```python
from build123d import *

# Parameters (mm, degrees)
BOSS_EXTRUDE1_DEPTH = 15
SKETCH2_R           = 7.490706033
BOSS_EXTRUDE2_DEPTH = 5
SKETCH3_R           = 8.44094948
BOSS_EXTRUDE3_DEPTH = 7
FILLET1_R           = 1


with BuildPart() as part:
    # Sketch1 → Boss-Extrude1 (new body)
    with BuildSketch(Plane(origin=(0, 0, 0), x_dir=(1, 0, 0), z_dir=(0, 1, 0))):
        with BuildLine():
            Line((-17.967290282, 0), (-45.431439127, 0))
            ThreePointArc((-45.431439127, 0), (-58.787226235, 13.355787108), (-45.431439127, 26.711574216))
            Line((-45.431439127, 26.711574216), (5.45092281, 18.253380544))
            ThreePointArc((5.45092281, 18.253380544), (25.659892843, 17.20031813), (45.593289448, 20.689029929))
            Line((45.593289448, 20.689029929), (45.940338636, 20.791055963))
            Line((45.940338636, 20.791055963), (45.352375673, 22.791055963))
            ThreePointArc((45.352375673, 22.791055963), (25.570805515, 18.868293737), (5.45092281, 20.242666786))
            Line((5.45092281, 20.242666786), (-45.495890395, 28.711574216))
            ThreePointArc((-45.495890395, 28.711574216), (-62.583598174, 18.547920568), (-55.423692083, 0))
            Line((-55.423692083, 0), (-125.431439127, 0))
            Line((-125.431439127, 0), (-157.707883989, -16.232049306))
            Line((-157.707883989, -16.232049306), (-156.809303927, -18.01882122))
            Line((-156.809303927, -18.01882122), (-124.532859065, -1.786771914))
            Line((-124.532859065, -1.786771914), (-17.068710221, -1.786771914))
            ThreePointArc((-17.068710221, -1.786771914), (1.299435065, -3.480980646), (19.190909572, -7.970328534))
            Line((19.190909572, -7.970328534), (30.410309542, -11.40707822))
            Line((30.410309542, -11.40707822), (30.996087081, -9.494785179))
            Line((30.996087081, -9.494785179), (17.179362085, -5.262417546))
            ThreePointArc((17.179362085, -5.262417546), (-0.198073846, -1.322896281), (-17.967290282, 0))
        make_face()
    extrude(amount=BOSS_EXTRUDE1_DEPTH)

    # Sketch2 → Boss-Extrude2 (add)
    with BuildSketch(Plane(origin=(-132.388101561, 0, 66.578899913), x_dir=(0.4492900307338926, 0, 0.8933859570662267), z_dir=(-0.8933859570662267, 0, 0.4492900307338926))):
        with Locations(Location((-55.356167213, 7.508040546, 0), (0, 0, 97.663545488))):
            Circle(SKETCH2_R)
    extrude(amount=BOSS_EXTRUDE2_DEPTH)

    # Sketch3 → Boss-Extrude3 (add)
    with BuildSketch(Plane(origin=(-136.855031347, 0, 68.825350067), x_dir=(0.4492900307338926, 0, 0.8933859570662267), z_dir=(-0.8933859570662267, 0, 0.4492900307338926))):
        with Locations((-55.356167213, 7.508040546)):
            Circle(SKETCH3_R)
    extrude(amount=BOSS_EXTRUDE3_DEPTH)

    # Fillet1
    fillet1_edges = [part.edges().sort_by_distance(p)[0] for p in [
        (-171.772141566, 7.508040546, 14.974932127),
    ]]
    fillet(fillet1_edges, radius=FILLET1_R)

    # Fillet3: read off the stored shape, not the designer's step
    # Fillet3 outline → Fillet3 (revolve, cut)
    with BuildSketch(Plane(origin=(-24.870974068, 7.508040546, -49.454422425), x_dir=(0.4492900307338924, 0, 0.8933859570662267), z_dir=(0, 1, 0))):
        with BuildLine():
            Line((8.44094948, -159.186906806), (8.44094948, -154.186906806))
            ThreePointArc((8.44094948, -154.186906806), (6.683590167, -158.429547493), (2.44094948, -160.186906806))
            Line((2.44094948, -160.186906806), (7.44094948, -160.186906806))
            ThreePointArc((7.44094948, -160.186906806), (8.148056261, -159.894013587), (8.44094948, -159.186906806))
        make_face()
    revolve(axis=Axis((-24.870974068, 7.508040546, -49.454422425), (0.8933859570662267, 0, -0.4492900307338924)), mode=Mode.SUBTRACT)


solid = part.part
```
Can you work these out from the model? Positions are in its coordinate system, mm. A direction names the side the tool comes from. Coordinates: 2 decimals unless noted, no trailing zeros. Loops run counter-clockwise (first coordinate to the right, second up) from the corner with the lowest first, then second, coordinate; pieces in that order, holes last.
1) Imagine slicing it at A-A on x = -24.5. List the corners of the cut face in (y, z) for me.
2) For pin 1 (6 mm diameter, centred on y = 11.5, z = 10.5, fed in from +X); pin 2 (1.5 mm diameter, centred on x = -123.5, y = 2, fed in from -Z); pin 3 (6 mm diameter, centred on x = -45, y = 12, fed in from +Z); pin 4 (23.5 mm diameter, centred on x = -87.5, z = -15.5, fed in from -Y), each with a flat end and sliding along its axis, tell me the tip position at first contact or that it passes through.
3) Which directions (+Z, -Z, +X, -X, +Y, -Y) give clear straight access to the entire face, cutting with the end or side of a thin tool? Please do faces 4 (the flat face through (-20.346, 7.395, -22.542)), 5 (the flat face through (-155.6, 7.77, 20.42)), 6 (the cylindrical face through (-156.1, 6.9, 24.9)), 7 (the flat face through (-167.995, 7.542, 22.485)), 8 (the flat face through (-141.34, 7.4, 8)).
4) I need wall thicknesses on probe 1 along Y at (x, z) = (-95, 1.5); probe 2 along Z at (x, y) = (-100.5, 4.5); probe 3 along Z at (x, y) = (23, 8.75). Which ranges of each line are inside material? Lowest first, please.
5) Imagine slicing it at B-B on x = -79. List the corners of the cut face in (y, z) for me, plus the area to 3 significant figures.
6) Thinking about a two-plate mould opening in Z: for faces 1 (the flat face through (24.722, 7.395, 9.665)), 2 (the flat face through (-158.95, 7.03, 13.76)), 3 (the cylindrical face through (25.376, 7.395, -17.184)), which applies, pulls with the +Z half, pulls with the -Z half, needs draft (parallel to the pull), parting line crosses it, or undercut?
Completed:
1. outline: (0, -25.22) - (15, -25.22) - (15, -23.23) - (0, -23.23) - close; (0, 0) - (15, 0) - (15, 1.79) - (0, 1.79) - close
2. pin 1: stops at x = 31
2. pin 2: stops at z = 0
2. pin 3: stops at z = 1.79
2. pin 4: passes through
3. face 4: +Y, -Y
3. face 5: +X, +Y, -Y
3. face 6: none
3. face 7: +Z, -X, +Y, -Y
3. face 8: -Z, +Y, -Y
4. probe 1: y = 0 to 15
4. probe 2: z = 0 to 1.79
4. probe 3: z = -18.75 to -17.08, 7.05 to 9.14
5. outline: (0, 0) - (15, 0) - (15, 1.79) - (0, 1.79) - close
5. area: 26.8 mm2
6. face 1: pulls with the +Z half
6. face 2: pulls with the -Z half
6. face 3: undercut
